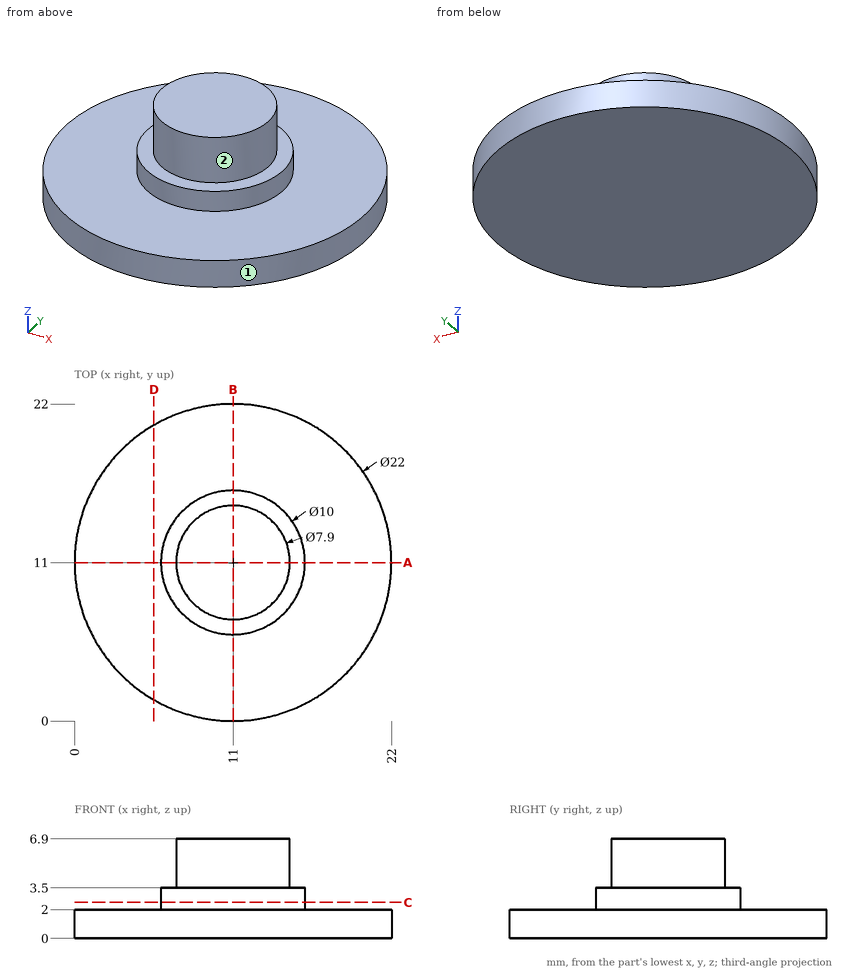
For this review, use the dimensioned drawing (mm, ordinates from the lowest corner) and the shaded views. A direction names the side the tool comes from. Round coordinates to 2 decimals unless told otherwise and drop trailing zeros. Write each loop counter-clockwise with the first axis right and the second up, starting at its lowest first coordinate (ties: lowest second). Pieces come first, ordered by that corner, then holes. Notation, with made-up numbers: M 46.25,78 L 69.25,78 A33 cw 69.25,109 Z; hole C 24,-11 d4. An arc over 180 degrees is marked long. Write item = value, one per line. Start each with the question number.
(1) Clearance check with flat-ended pins moving along their axes: pin 1 Ø12 at (x, y) = (11.5, 13.5) entering from -Z; pin 2 Ø4 at (y, z) = (14, 1.5) entering from -X; pin 3 Ø2 at (y, z) = (9.5, 5) entering from -X; pin 4 Ø3 at (x, y) = (17, 12) entering from +Z. State where each tip first meets the part, or that it passes through.
(2) For line 1 along Z through (x, y) = (14, 16.75); line 2 along X through (y, z) = (3.75, 1.75); line 3 along X through (y, z) = (6.25, 1.75), list the stretches that pass through material, from the lowest coordinate up.
(3) We need section A-A (y = 11). Give the boundary of the cut face in (x, z).
(4) We need section D-D (x = 5.5). Give the boundary of the cut face in (y, z), then the cut area to 3 significant figures.
(5) For the marked faces 1 and 2, list the 3-axis set-ups (+Z, -Z, +X, -X, +Y, -Y) from which the entire face can be reached by the end or side of a thin tool; tool diameter is ignored.
(6) We need section C-C (z = 2.5). Give the boundary of the cut face in (x, y), then the cut area to 3 significant figures.
Results found:
q1.pin_1 = 0
q1.pin_2 = 0.05
q1.pin_3 = 7.08
q1.pin_4 = 3.5
q2.line_1 = 0 to 2
q2.line_2 = 2.73 to 19.27
q2.line_3 = 1.08 to 20.92
q3.outline = M 0,0 L 22,0 L 22,2 L 16,2 L 16,3.5 L 14.95,3.5 L 14.95,6.9 L 7.05,6.9 L 7.05,3.5 L 6,3.5 L 6,2 L 0,2 Z
q4.outline = M 1.47,0 L 20.53,0 L 20.53,2 L 1.47,2 Z
q4.area = 38.1 mm²
q5.face_1 = +Z, -Z
q5.face_2 = +Z
q6.outline = C 11,11 d10
q6.area = 78.5 mm²
